Can you work these out from the model? Positions are in its coordinate system, mm. A direction names the side the tool comes from. Round coordinates to 2 decimals unless told otherwise and drop trailing zeros. Loops run counter-clockwise (first coordinate to the right, second up) from the corner with the lowest first, then second, coordinate; pieces in that order, holes last.
(1) Thinking about a two-plate mould opening in Z: for faces 3 (the face through (1.81, 6.51, -147.99)), 4 (the face through (112.521, 74.982, 1.635)), 5 (the face through (114, 78, 0)), which applies, released by +Z, released by -Z, zero draft, split by the parting line, or undercut?
(2) I want a section at D-D on x = -16. Write out the boundary of the cut face in (y, z).
(3) Which directions (+Z, -Z, +X, -X, +Y, -Y) give clear straight access to the entire face, cutting with the end or side of a thin tool? Please do faces 1 (the face through (-1.77, 6.6, 144.99)), 2 (the face through (-112.479, 74.982, -1.635)).
(4) Will these pins go through, and if not, where does the flat tip stop? pin 1 Ø6 at (y, z) = (69, -91) entering from -X; pin 2 Ø4 at (x, z) = (64, 12) entering from +Y; pin 3 Ø1 at (x, y) = (72, 115) entering from +Z.
(5) I want a section at C-C on y = 114.5. Write out the boundary of the cut face in (x, z) (1 decimal), plus the area to 3 significant figures.
(6) I want a section at A-A on z = 0. Write out the boundary of the cut face in (x, y).
(7) I want a section at B-B on x = 32.5. Write out the boundary of the cut face in (y, z).
(8) If I drill on line 1 along X through (y, z) = (16.5, -73.5); line 2 along Z through (x, y) = (80.5, 46.5); line 3 along Z through (x, y) = (-12.5, 45), over which ranges is the centre line in solid material (lowest first)?
from build123d import *

# Parameters (mm, degrees)
ESQUISSE2_OUTSIDE_W     = 386.766
ESQUISSE2_OUTSIDE_H     = 238.266
ESQUISSE2_OUTSIDE_W_2   = 228
ESQUISSE2_OUTSIDE_H_2   = 155
ENL_V_MAT_EXTRU_1_DEPTH = 150
BOSS_EXTRU_1_DEPTH      = 3
BOSS_EXTRU_2_START      = -3
BOSS_EXTRU_2_DEPTH      = 3
CONG_1_R                = 3


with BuildPart() as part:
    # Esquisse1 → Révolution4 (revolve)
    with BuildSketch(Plane.XY, mode=Mode.PRIVATE) as r_volution4_sk:
        with BuildLine():
            Line((148, 12.175795662), (148, 1))
            Line((148, 1), (145, 1))
            Line((145, 1), (145, 12.051970793))
            ThreePointArc((145, 12.051970793), (98.530929788, 107.060290842), (0, 145.5))
            Line((0, 145.5), (0, 148.5))
            ThreePointArc((0, 148.5), (100.608509442, 109.225353412), (148, 12.175795662))
        make_face()
    revolve(r_volution4_sk.sketch.rotate(Axis((0, 0, 0), (0, 1, 0)), 90), axis=Axis((0, 0, 0), (0, 1, 0)))

    # Esquisse2 outside → Enlèv. mat.-Extru.1 (cut, symmetric)
    with BuildSketch(Plane.XY):
        with Locations((0, 74.75)):
            Rectangle(ESQUISSE2_OUTSIDE_W, ESQUISSE2_OUTSIDE_H)
        with Locations((0, 72.5)):
            Rectangle(ESQUISSE2_OUTSIDE_W_2, ESQUISSE2_OUTSIDE_H_2, mode=Mode.SUBTRACT)
    extrude(amount=ENL_V_MAT_EXTRU_1_DEPTH, both=True, mode=Mode.SUBTRACT)

    # Esquisse3 → Boss.-Extru.1 (add)
    with BuildSketch(Plane(origin=(114, 0, 0), x_dir=(0, 0, -1), z_dir=(1, 0, 0))):
        with BuildLine():
            Line((-93.994680701, 1), (-74.993333037, 1))
            ThreePointArc((-74.993333037, 1), (0, 75), (74.993333037, 1))
            Line((74.993333037, 1), (93.994680701, 1))
            ThreePointArc((93.994680701, 1), (0, 94), (-93.994680701, 1))
        make_face()
    extrude(amount=-BOSS_EXTRU_1_DEPTH)

    # Esquisse4 → Boss.-Extru.2 (add)
    with BuildSketch(Plane.ZY.offset(114).offset(BOSS_EXTRU_2_START)):
        with BuildLine():
            Line((-93.994680701, 1), (-74.993333037, 1))
            ThreePointArc((-74.993333037, 1), (0, 75), (74.993333037, 1))
            Line((74.993333037, 1), (93.994680701, 1))
            ThreePointArc((93.994680701, 1), (0, 94), (-93.994680701, 1))
        make_face()
    extrude(amount=BOSS_EXTRU_2_DEPTH)

    # Congé1
    # the kernel refuses this fillet: 3 mm, written as the material it takes off along each edge
    with BuildSketch(Plane(origin=(-114, 20.411983352, -94.382201712), x_dir=(0.6405708887604551, 0, -0.767899040546764), z_dir=(0, -1, 0)), Plane(origin=(114, 20.411983352, 94.382201712), x_dir=(-0.6405708887604538, 0, 0.7678990405467649), z_dir=(0, -1, 0))) as cong_1_piece_1:
        with BuildLine():
            CenterArc((1.087028375, 2.999979354), CONG_1_R, 230.165597581, 40.046969931)
            Line((-0.834684291, 0.696282232), (0, 0))
            ThreePointArc((0, 0), (0.549079179, -0.001018544), (1.098158359, 0))
        make_face()
    extrude(amount=22.157379249, mode=Mode.SUBTRACT)
    with BuildSketch(Plane(origin=(-114, 0, 0), x_dir=(0, 0.09906318090270165, -0.9950811455300712), z_dir=(0, -0.9950811455300712, -0.09906318090270165))) as cong_1_piece_2:
        with BuildLine():
            CenterArc((94.070452322, 3), CONG_1_R, 270, 40.28066089)
            ThreePointArc((96.010049277, 0.711340206), (95.587852119, 0.354883399), (95.164331553, 0))
            Line((95.164331553, 0), (94.070452322, 0))
        make_face()
    revolve(axis=Axis((-114, 0, 0), (1, 0, 0)), revolution_arc=168.629546335, mode=Mode.SUBTRACT)
    with BuildSketch(Plane(origin=(-114, 20.411983352, 94.382201712), x_dir=(0, 0, -1), z_dir=(0, -1, 0))) as cong_1_piece_3:
        with BuildLine():
            CenterArc((1.086971394, 3), CONG_1_R, 229.953030069, 40.046969931)
            ThreePointArc((-0.84327475, 0.703448276), (-0.422289825, 0.350941999), (0, 0))
            Line((0, 0), (1.086971394, 0))
        make_face()
    extrude(amount=22.157379249, mode=Mode.SUBTRACT)
    with BuildSketch(Plane(origin=(114, 0, 0), x_dir=(0, 0.09906318090270108, 0.9950811455300712), z_dir=(0, -0.9950811455300712, 0.09906318090270108))) as cong_1_piece_4:
        with BuildLine():
            CenterArc((94.070452322, 3), CONG_1_R, 270, 40.28066089)
            Line((94.070452322, 0), (95.164331553, 0))
            ThreePointArc((95.164331553, 0), (95.587852119, 0.354883399), (96.010049277, 0.711340206))
        make_face()
    revolve(axis=Axis((114, 0, 0), (-1, 0, 0)), revolution_arc=168.629546335, mode=Mode.SUBTRACT)
    with BuildSketch(Plane(origin=(114, 20.411983352, -94.382201712), x_dir=(-0.6405708887604424, 0, -0.7678990405467746), z_dir=(0, -1, 0))) as cong_1_piece_5:
        with BuildLine():
            CenterArc((1.087028375, -2.999979354), CONG_1_R, 89.787432488, 40.046969931)
            Line((-0.834684291, -0.696282232), (0, 0))
            ThreePointArc((0, 0), (0.549079179, 0.001018544), (1.098158359, 0))
        make_face()
    extrude(amount=22.157379249, mode=Mode.SUBTRACT)


solid = part.part
Filled sheet:
1. face 3: released by -Z
1. face 4: undercut
1. face 5: zero draft
2. outline: (1, -147.13) - (12.18, -147.13) arc R147.64 ccw to (12.18, 147.13) - (1, 147.13) - (1, 144.11) - (12.05, 144.11) arc R144.62 cw to (12.05, -144.11) - (1, -144.11) - close
3. face 1: -Y
3. face 2: +X, -X, -Y
4. pin 1: stops at x = -98.42
4. pin 2: stops at y = 134.42
4. pin 3: stops at z = 61.47
5. outline: circle Ø189.1 at (0, 0); hole circle Ø179.6 at (0, 0)
5. area: 2,770 mm2
6. outline: (-114, 75) - (-111, 75) - (-111, 94) - (-111.06, 94) arc R145.5 cw to (111.06, 94) - (111, 94) - (111, 75) - (114, 75) - (114, 94.07) arc R3 ccw to (113.29, 96.01) arc R148.5 ccw to (-113.29, 96.01) arc R3 ccw to (-114, 94.07) - close
7. outline: (1, -144.39) - (12.18, -144.39) arc R144.9 ccw to (12.18, 144.39) - (1, 144.39) - (1, 141.31) - (12.05, 141.31) arc R141.82 cw to (12.05, -141.31) - (1, -141.31) - close
8. line 1: x = -114 to -111, 111 to 114
8. line 2: z = -115.8 to -111.93, 111.93 to 115.8
8. line 3: z = -140.96 to -137.8, 137.8 to 140.96
